Check sheet for the modelled part. Datum: model origin and axes. Units: mm. Face numbers are marked on the shaded views. A direction names the side the tool comes from. Coordinates: 2 decimals unless noted, no trailing zeros. Loops run counter-clockwise (first coordinate to the right, second up) from the corner with the lowest first, then second, coordinate; pieces in that order, holes last. Notation, with made-up numbers: (-25, -3.75) -> (7, -3.75) arc R17 cw to (7, 24.25) -> close; hole circle Ø4 at (24.25, -27). An arc over 180 degrees is marked (long way). Use CSV: the item, a comma, the result in double quotes.
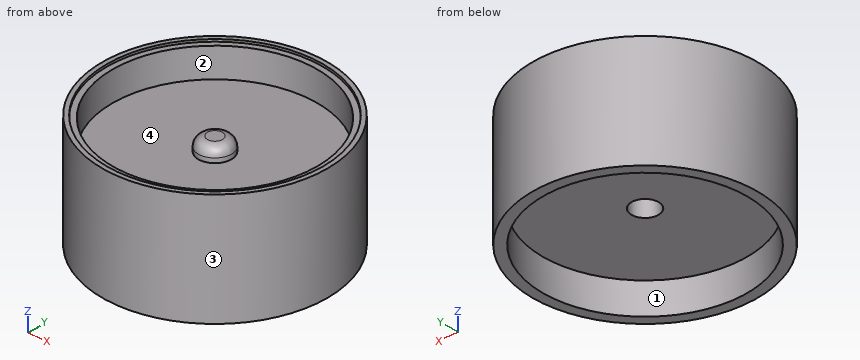
Autodesk Inventor part; units mm, degrees
ref_plane "YZ Plane" through (0, 0, 0) normal (1, 0, 0) x (0, 1, 0)
ref_plane "XZ Plane" through (0, 0, 0) normal (0, 1, 0) x (-1, 0, 0)
ref_plane "XY Plane" through (0, 0, 0) normal (0, 0, 1) x (1, 0, 0)
sketch "Sketch1" plane through (0, 0, 0) normal (0, 0, 1) x (1, 0, 0)
  circle A0 centre (0, 0) radius 25
  dimension "d0" = 50
extrude "Extrusion1" add sketch "Sketch1" along normal blind 25
sketch "Sketch2" plane through (0, 0, 25) normal (0, 0, 1) x (1, 0, 0)
  circle A0 centre (0, 0) radius 22.7546
sketch "Sketch3" plane through (0, 0, 0) normal (0, 0, -1) x (-1, 0, 0)
  circle A0 centre (0, 0) radius 22.7077
extrude "Extrusion2" cut sketch "Sketch2" against normal blind 7
extrude "Extrusion3" cut sketch "Sketch3" against normal blind 7
sketch "Sketch4" plane through (0, 0, 25) normal (0, 0, 1) x (1, 0, 0)
  circle A0 centre (0, 0) radius 24.0163
extrude "Extrusion4" cut sketch "Sketch4" against normal blind 0.5
sketch "Sketch5" plane through (0, 0, 18) normal (0, 0, 1) x (1, 0, 0)
  circle A0 centre (0, 0) radius 3
  dimension "d9" = 6
extrude "Extrusion5" cut sketch "Sketch5" against normal blind 25
sketch "Sketch6" plane through (0, 0, 18) normal (0, 0, 1) x (1, 0, 0)
  circle A0 centre (0, 0) radius 3.6832
extrude "Extrusion6" add sketch "Sketch6" along normal blind 3
fillet "Fillet1" radius 2 1 edges at (-3.6832, 0, 21)
sketch "Sketch7" plane through (0, 0, 18) normal (0, 0, 1) x (1, 0, 0)
  point P0 (0, 0)
sketch "Sketch8" plane through (0, 0, 18) normal (0, 0, 1) x (1, 0, 0)
  point P0 (0, 0)
properties part number "WHEEL 2"
1) Access from +Z, -Z, +X, -X, +Y, -Y to the whole of each face (thin tool, end or side, straight path). Record for the marked faces 1 and 2.
Answer below:
face 1,"-Z"
face 2,"+Z"
2) Cross-section at A-A on z = 13. Record the boundary of the cut face in (x, y), and give its area (3 significant figures).
Answer below:
outline,"circle Ø50 at (0, 0); hole circle Ø6 at (0, 0)"
area,"1,940 mm²"
3) Cross-section at D-D on z = 5.25. Record the boundary of the cut face in (x, y).
Answer below:
outline,"circle Ø50 at (0, 0); hole circle Ø45.42 at (0, 0)"
4) Go/stop test with flat-tipped pins: pin 1 Ø4 at (x, z) = (-19, 12.5) entering from +Y; pin 2 Ø3.5 at (x, y) = (0, 0) entering from +Z; pin 3 Ø3 at (x, z) = (6.5, 11.5) entering from -Y. Record where each tip stops, or that it passes through.
Answer below:
pin 1,"stops at y = 18.33"
pin 2,"stops at z = 21"
pin 3,"stops at y = -24.49"
5) Thickness scan on line 1 along Y through (x, z) = (0, 20.5); line 2 along Y through (x, z) = (0, 1.5); line 3 along Y through (x, z) = (0, 22). Record the ranges inside material, lowest first. Write a range as from..to.
Answer below:
line 1,"y = -25..-22.75, -3.01..3.01, 22.75..25"
line 2,"y = -25..-22.71, 22.71..25"
line 3,"y = -25..-22.75, 22.75..25"
6) Cross-section at C-C on x = 7. Record the boundary of the cut face in (y, z).
Answer below:
outline,"(-24, 0) -> (-21.6, 0) -> (-21.6, 7) -> (21.6, 7) -> (21.6, 0) -> (24, 0) -> (24, 25) -> (22.97, 25) -> (22.97, 24.5) -> (21.65, 24.5) -> (21.65, 18) -> (-21.65, 18) -> (-21.65, 24.5) -> (-22.97, 24.5) -> (-22.97, 25) -> (-24, 25) -> close"
7) Draft check along Y on the marked faces 3 and 4. Enter one of: released by +Y, released by -Y, zero draft, split by the parting line, or undercut.
Answer below:
face 3,"split by the parting line"
face 4,"undercut"
8) Cross-section at B-B on y = -21. Record the boundary of the cut face in (x, z).
Answer below:
outline,"(-13.56, 0) -> (-8.64, 0) -> (-8.64, 7) -> (8.64, 7) -> (8.64, 0) -> (13.56, 0) -> (13.56, 25) -> (11.65, 25) -> (11.65, 24.5) -> (8.76, 24.5) -> (8.76, 18) -> (-8.76, 18) -> (-8.76, 24.5) -> (-11.65, 24.5) -> (-11.65, 25) -> (-13.56, 25) -> close"
